For this review, take the finished solid that the model builds, in its own axes (mm). Face numbers are marked on the shaded views. A direction names the side the tool comes from. Round coordinates to 2 decimals unless told otherwise and drop trailing zeros. Write each loop counter-clockwise with the first axis right and the second up, starting at its lowest first coordinate (ties: lowest second). Pieces come first, ordered by that corner, then holes.
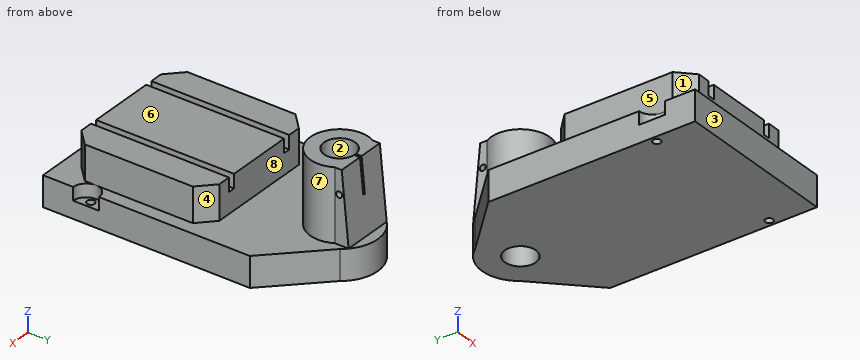
from build123d import *

# Parameters (mm, degrees)
F0_R      = 4.5
F1_DEPTH  = 35
F2_DEPTH  = 24
F3_DEPTH  = 15
F5_DEPTH  = 35
F7_DEPTH  = 83
F9_DEPTH  = 125
F10_R     = 18
F11_DEPTH = 222
F12_W     = 2.5
F12_H     = 32
F13_DEPTH = 40
F8_R      = 3.5
F14_DEPTH = 94.3
F15_W     = 78
F15_H     = 160
F16_DEPTH = 16
F17_DEPTH = 24


with BuildPart() as f1:
    # F0 (on Top) → F1 (new body)
    with BuildSketch(Plane.XY):
        with BuildLine():
            Line((35, 160), (-35, 160))
            Line((-35, 160), (-95, 100))
            Line((-95, 100), (-95, -75))
            ThreePointArc((-95, -75), (-84.3933982822, -79.3933982822), (-80, -90))
            Line((-80, -90), (-80, 40))
            Line((-80, 40), (80, 40))
            Line((80, 40), (80, -90))
            ThreePointArc((80, -90), (84.3933982822, -79.3933982822), (95, -75))
            Line((95, -75), (95, 100))
            Line((95, 100), (35, 160))
        make_face()
        Polygon((-80, 40), (-80, -90), (-80, -120), (80, -120), (80, -90), (80, 40), align=None)
        with BuildLine():
            ThreePointArc((-80, -90), (-84.3933982822, -100.6066017178), (-95, -105))
            Line((-95, -105), (-95, -140))
            Line((-95, -140), (95, -140))
            Line((95, -140), (95, -105))
            ThreePointArc((95, -105), (84.3933982822, -100.6066017178), (80, -90))
            Line((80, -90), (80, -120))
            Line((80, -120), (-80, -120))
            Line((-80, -120), (-80, -90))
        make_face()
        with BuildLine():
            Line((95, -105), (95, -75))
            ThreePointArc((95, -75), (84.3933982822, -79.3933982822), (80, -90))
            ThreePointArc((80, -90), (84.3933982822, -100.6066017178), (95, -105))
        make_face()
        with Locations((87.5, -90)):
            Circle(F0_R, mode=Mode.SUBTRACT)
        with BuildLine():
            ThreePointArc((-80, -90), (-84.3933982822, -79.3933982822), (-95, -75))
            Line((-95, -75), (-95, -105))
            ThreePointArc((-95, -105), (-84.3933982822, -100.6066017178), (-80, -90))
        make_face()
        with Locations((-87.5, -90)):
            Circle(F0_R, mode=Mode.SUBTRACT)
    extrude(amount=-F1_DEPTH)

    # F0 (on Top) → F2 (join)
    with BuildSketch(Plane.XY):
        Polygon((-80, 40), (-80, -90), (-80, -120), (80, -120), (80, -90), (80, 40), align=None)
    extrude(amount=F2_DEPTH)

    # F0 (on Top) → F3 (cut)
    with BuildSketch(Plane.XY):
        with BuildLine():
            ThreePointArc((-80, -90), (-84.3933982822, -79.3933982822), (-95, -75))
            Line((-95, -75), (-95, -105))
            ThreePointArc((-95, -105), (-84.3933982822, -100.6066017178), (-80, -90))
        make_face()
        with Locations((-87.5, -90)):
            Circle(F0_R, mode=Mode.SUBTRACT)
        with BuildLine():
            Line((95, -105), (95, -75))
            ThreePointArc((95, -75), (84.3933982822, -79.3933982822), (80, -90))
            ThreePointArc((80, -90), (84.3933982822, -100.6066017178), (95, -105))
        make_face()
        with Locations((87.5, -90)):
            Circle(F0_R, mode=Mode.SUBTRACT)
    extrude(amount=-F3_DEPTH, mode=Mode.SUBTRACT)

    # F4 (on face) → F5 (join)
    with BuildSketch(Plane.XY):
        with BuildLine():
            Line((-35, 160), (35, 160))
            ThreePointArc((35, 160), (0, 177.7706570637), (-35, 160))
        make_face()
    extrude(amount=-F5_DEPTH)

    # F6 (on face) → F7 (join)
    with BuildSketch(Plane.XY):
        with BuildLine():
            Line((29.6988346186, 166), (-29.6988346186, 166))
            Line((-29.6988346186, 166), (-29.6988346186, 150))
            ThreePointArc((-29.6988346186, 150), (0, 99.4476822681), (29.6988346186, 150))
            Line((29.6988346186, 150), (29.6988346186, 166))
        make_face()
    extrude(amount=F7_DEPTH)

    # F8 (on face) → F9 (cut)
    with BuildSketch(Plane.YZ.offset(29.6988346186)):
        Polygon((158, 83), (166, 0), (166, 83), align=None)
    extrude(amount=-F9_DEPTH, mode=Mode.SUBTRACT)

    # F10 (on face) → F11 (cut)
    with BuildSketch(Plane.XY.offset(83)):
        with Locations((0, 133.4476822681)):
            Circle(F10_R)
    extrude(amount=-F11_DEPTH, mode=Mode.SUBTRACT)

    # F12 (on face) → F13 (cut)
    with BuildSketch(Plane.XY.offset(83)):
        with Locations((0, 174)):
            Rectangle(F12_W, F12_H)
        with BuildLine():
            Line((1.25, 158), (-1.25, 158))
            Line((-1.25, 158), (-1.25, 151.404227036))
            ThreePointArc((-1.25, 151.404227036), (0, 151.4476822681), (1.25, 151.404227036))
            Line((1.25, 151.404227036), (1.25, 158))
        make_face()
        with BuildLine():
            ThreePointArc((1.25, 151.404227036), (0, 151.4476822681), (-1.25, 151.404227036))
            Line((-1.25, 151.404227036), (-1.25, 140))
            Line((-1.25, 140), (1.25, 140))
            Line((1.25, 140), (1.25, 151.404227036))
        make_face()
    extrude(amount=-F13_DEPTH, mode=Mode.SUBTRACT)

    # F8 (on face) → F14 (cut)
    with BuildSketch(Plane.YZ.offset(29.6988346186)):
        with Locations((155, 55)):
            Circle(F8_R)
    extrude(amount=-F14_DEPTH, mode=Mode.SUBTRACT)

    # F15 (on face) → F16 (join)
    with BuildSketch(Plane.XY.offset(24)):
        Polygon((62, 40), (47, 40), (47, -120), (62, -120), (80, -102.6506484271), (80, 22.6506484271), align=None)
        with Locations((0, -40)):
            Rectangle(F15_W, F15_H)
        Polygon((-47, -120), (-47, 40), (-62, 40), (-80, 22.6506484271), (-80, -102.6506484271), (-62, -120), align=None)
    extrude(amount=F16_DEPTH)

    # F17 (cut): faces of the model
    f17_faces = [f1.faces().sort_by_distance(p)[0] for p in [
        (-74, 34.216882809, 24),
        (-74, -114.216882809, 24),
        (74, -114.216882809, 24),
        (74, 34.216882809, 24),
    ]]
    extrude(f17_faces, amount=-F17_DEPTH, mode=Mode.SUBTRACT)


solid = f1.part
(1) Mouldability with a two-part tool opening along X and no side actions: class the marked faces 1, 2, 3 and 4 as pulls with the +X half, pulls with the -X half, needs draft (parallel to the pull), parting line crosses it, or undercut.
Geometry check:
face 1: pulls with the -X half
face 2: undercut
face 3: needs draft
face 4: pulls with the +X half
(2) We need section A-A, the plane z = 28. Give the boundary of the cut face in (x, y).
Geometry check:
outline: (-80, -102.65) - (-62, -120) - (-47, -120) - (-47, 40) - (-62, 40) - (-80, 22.65) - close; (-39, -120) - (39, -120) - (39, 40) - (-39, 40) - close; (-29.7, 150) arc R34 ccw (long way) to (29.7, 150) - (29.7, 163.3) - (-29.7, 163.3) - close; (47, -120) - (62, -120) - (80, -102.65) - (80, 22.65) - (62, 40) - (47, 40) - close; hole circle Ø36 at (0, 133.45)
(3) For line 1 along X through (y, z) = (-90, 27); line 2 along X through (y, z) = (134.5, 76); line 3 along Z through (x, y) = (-12, 155), list the stretches that pass through material, from the lowest coordinate up.
Geometry check:
line 1: x = -80 to -47, -39 to 39, 47 to 80
line 2: x = -33.98 to -17.97, 17.97 to 33.98
line 3: z = -35 to 51.5, 58.5 to 83
(4) For pin 1 Ø3 at (y, z) = (156.5, 57) entering from -X; pin 2 Ø1.3 at (x, y) = (0, 154.5) entering from +Z; pin 3 Ø3 at (x, z) = (-30.5, 18) entering from +Y; pin 4 Ø5.5 at (x, y) = (-87.5, -90) entering from -Z, all flat-tipped, find the tip position at first contact; note any pin that passes through.
Geometry check:
pin 1: stops at x = -29.7
pin 2: stops at z = 43
pin 3: stops at y = 164.39
pin 4: passes through
(5) We need section B-B, the plane x = 52.5. Give the boundary of the cut face in (y, z).
Geometry check:
outline: (-140, -35) - (142.5, -35) - (142.5, 0) - (40, 0) - (40, 40) - (-120, 40) - (-120, 0) - (-140, 0) - close
(6) We need section D-D, the plane x = -11. Give the boundary of the cut face in (y, z).
Geometry check:
outline: (-140, -35) - (119.2, -35) - (119.2, 83) - (101.28, 83) - (101.28, 0) - (40, 0) - (40, 40) - (-120, 40) - (-120, 0) - (-140, 0) - close; (147.7, -35) - (176.35, -35) - (176.35, 0) - (166, 0) - (158, 83) - (147.7, 83) - close; hole circle Ø7 at (155, 55)
(7) For the marked faces 5, 6, 7 and 8, list the 3-axis set-ups (+Z, -Z, +X, -X, +Y, -Y) from which the entire face can be reached by the end or side of a thin tool; tool diameter is ignored.
Geometry check:
face 5: +Z, -X, +Y, -Y
face 6: +Z, +X, -X, -Y
face 7: +Z
face 8: +Z, +X, -X
(8) We need section C-C, the plane y = -71. Give the boundary of the cut face in (x, z).
Geometry check:
outline: (-95, -35) - (95, -35) - (95, 0) - (80, 0) - (80, 40) - (47, 40) - (47, 24) - (39, 24) - (39, 40) - (-39, 40) - (-39, 24) - (-47, 24) - (-47, 40) - (-80, 40) - (-80, 0) - (-95, 0) - close
